Source: CAD feature listing. Evaluate the final solid. Frame: model axes, mm. Give positions to 0.01 mm unless a question says otherwise; leave off trailing zeros. Order: outer loops, then holes, each group sorted by start corner. A loop starts at its lowest first (then second) coordinate and runs counter-clockwise, first axis right, second up. Notation, with made-up numbers: M 33,76 L 38,76 A14 cw 38,102 Z; hole C 42,80.5 d5. An arc over 180 degrees is marked long. Use CSV: the item, a comma, the result in double quotes. Start each with the question number.
Item 1: Ray query, probe 1 along Y at (x, z) = (-7, 49); probe 2 along Z at (x, y) = (3, 5.5); probe 3 along X at (y, z) = (40, 61). Return the intervals inside material, ascending. Write a range as from..to.
Item 2: Section query D-D on x = -14. Return loops of the section in (y, z).
Item 3: First-contact query: pin 1 (12 mm diameter, centred on x = 0, z = 19.5, fed in from +Y); pin 2 (6 mm diameter, centred on x = -9, y = 7.5, fed in from -Z); pin 3 (10 mm diameter, centred on x = -7.5, y = 15.5, fed in from -Z). Flat tips, straight axial feed; report the tip coordinate or a pass-through.
Item 4: Section query C-C on y = 4. Return loops of the section in (x, z).
Item 5: Section query B-B on x = -1.5. Return loops of the section in (y, z), and give its area (3 significant figures).
Item 6: Section query A-A on z = 55. Return loops of the section in (x, y), and give its area (3 significant figures).
from build123d import *


with BuildPart() as f2:
    # F2: sweep along a path in F1
    with BuildLine(Plane.YZ) as f2_path:
        Line((0, 0), (42.337261, 32.216601))
    # F0 (on Front) → F2 (sweep)
    with BuildSketch(Plane.XZ):
        Polygon((-15.846774, 0), (0, 0), (15.846774, 0), (15.846774, 25.887098), (10.766129, 39.193552), (3.750001, 39.193552), (-3.750001, 39.193552), (-10.766129, 39.193552), (-15.846774, 25.887098), align=None)
    sweep(path=f2_path.line)


solid = f2.part
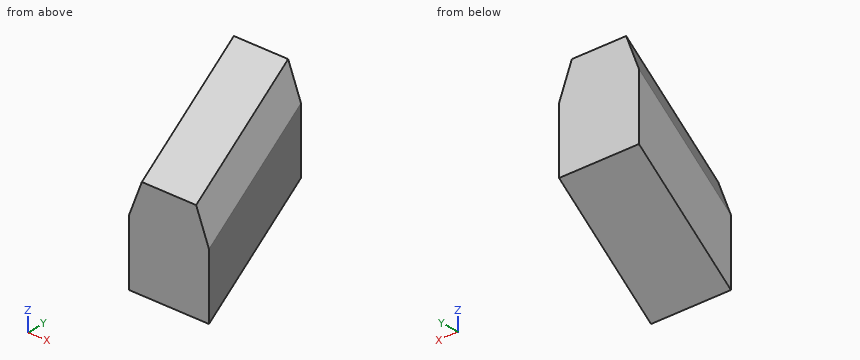
Verdict:
1,probe 1,"12.89..42.34"
1,probe 2,"4.19..43.38"
1,probe 3,"-14.06..14.06"
2,outline,"M 0,0 L 42.34,32.22 L 42.34,62.94 L 0,30.72 Z"
3,pin 1,"y = 33.51"
3,pin 2,"z = 3.42"
3,pin 3,"z = 7.99"
4,outline,"M -15.85,3.04 L 15.85,3.04 L 15.85,28.93 L 10.77,42.24 L -10.77,42.24 L -15.85,28.93 Z"
5,outline,"M 0,0 L 42.34,32.22 L 42.34,71.41 L 0,39.19 Z"
5,area,"1,660 mm2"
6,outline,"M -15.85,38.26 L -10.77,20.77 L 10.77,20.77 L 15.85,38.26 L 15.85,42.34 L -15.85,42.34 Z"
6,area,"595 mm2"
